from build123d import *

# Parameters (mm, degrees)
F0_W      = 127
F0_H      = 63.5
F1_DEPTH  = 177.8
F2_R      = 50.8
F3_DEPTH  = 101.6
F5_DEPTH  = 63.5
F6_R      = 19.05
F7_DEPTH  = 25.4
F9_DEPTH  = 38.1
F11_DEPTH = 38.1


with BuildPart() as f1:
    # F0 (on Front) → F1 (new body)
    with BuildSketch(Plane.XZ):
        with Locations((-4.952263087, -14.3639492443)):
            Rectangle(F0_W, F0_H)
    extrude(amount=F1_DEPTH)

    # F2 (on face) → F3 (join)
    with BuildSketch(Plane.XY.offset(17.3860507557)):
        with Locations((-4.952263087, -88.9)):
            Circle(F2_R)
    extrude(amount=F3_DEPTH)

    # F4 (on face) → F5 (cut)
    with BuildSketch(Plane.XY.offset(118.9860507557)):
        with BuildLine():
            ThreePointArc((-4.952263087, -38.1), (-30.352263087, -44.9059094878), (-48.9463535993, -63.5))
            ThreePointArc((-48.9463535993, -63.5), (-20.5993083432, -61.7985226281), (-4.952263087, -38.1))
        make_face()
        with BuildLine():
            ThreePointArc((39.0418274252, -63.5), (20.447736913, -44.9059094878), (-4.952263087, -38.1))
            ThreePointArc((-4.952263087, -38.1), (10.6947821691, -61.7985226281), (39.0418274252, -63.5))
        make_face()
        with BuildLine():
            ThreePointArc((45.847736913, -88.9), (44.1167688885, -75.7519925088), (39.0418274252, -63.5))
            ThreePointArc((39.0418274252, -63.5), (26.3418274252, -88.9), (39.0418274252, -114.3))
            ThreePointArc((39.0418274252, -114.3), (44.1167688885, -102.0480074912), (45.847736913, -88.9))
        make_face()
        with BuildLine():
            ThreePointArc((39.0418274252, -114.3), (10.6947821691, -116.0014773719), (-4.952263087, -139.7))
            ThreePointArc((-4.952263087, -139.7), (20.447736913, -132.8940905122), (39.0418274252, -114.3))
        make_face()
        with BuildLine():
            ThreePointArc((-4.952263087, -139.7), (-20.5993083432, -116.0014773719), (-48.9463535993, -114.3))
            ThreePointArc((-48.9463535993, -114.3), (-30.352263087, -132.8940905122), (-4.952263087, -139.7))
        make_face()
        with BuildLine():
            ThreePointArc((-48.9463535993, -114.3), (-36.2463535993, -88.9), (-48.9463535993, -63.5))
            ThreePointArc((-48.9463535993, -63.5), (-55.752263087, -88.9), (-48.9463535993, -114.3))
        make_face()
    extrude(amount=-F5_DEPTH, mode=Mode.SUBTRACT)

    # F6 (on face) → F7 (cut)
    with BuildSketch(Plane.XY.offset(118.9860507557)):
        with Locations((-4.952263087, -88.9)):
            Circle(F6_R)
    extrude(amount=-F7_DEPTH, mode=Mode.SUBTRACT)

    # F8 (on face) → F9 (cut)
    with BuildSketch(Plane.XY.offset(55.4860507557)):
        with BuildLine():
            ThreePointArc((-4.952263087, -139.7), (20.447736913, -132.8940905122), (39.0418274252, -114.3))
            ThreePointArc((39.0418274252, -114.3), (10.6947821691, -116.0014773719), (-4.952263087, -139.7))
        make_face()
    extrude(amount=-F9_DEPTH, mode=Mode.SUBTRACT)

    # F10 (on face) → F11 (cut)
    with BuildSketch(Plane.XY.offset(55.4860507557)):
        with BuildLine():
            Line((-4.952263087, -38.1), (39.0418274252, -63.5))
            ThreePointArc((39.0418274252, -63.5), (20.447736913, -44.9059094878), (-4.952263087, -38.1))
        make_face()
    extrude(amount=-F11_DEPTH, mode=Mode.SUBTRACT)


solid = f1.part
Could you check a few things on this model? Use its own coordinates, in mm. A direction names the side the tool comes from. Coordinates: 2 decimals unless noted, no trailing zeros. Loops run counter-clockwise (first coordinate to the right, second up) from the corner with the lowest first, then second, coordinate; pieces in that order, holes last.
1. Imagine slicing it at C-C (z = 46.5). Please give me the cut outline in (x, y), and give its area (3 significant figures).
2. For faces 5 (the face through (-20.958, -62.002, 87.681)), 6 (the face through (-36.25, -89.31, 87.68)), 7 (the face through (36, -89, 55.486)), which set-ups out of +Z, -Z, +X, -X, +Y, -Y let a thin tool reach every point of the face, with its end or its side?
3. For P1, Ø3, axis at x = -41, z = 50, coming from the -Y side; P2, Ø21.5, axis at x = -49.5, y = -92.5, coming from the +Z side; P3, Ø4, axis at x = 4, y = -88, coming from the +Z side, each with a flat end and sliding along its axis, tell me the tip position at first contact or that it passes through.
4. We'd pull the mould along X, two halves only. Please class faces 1 (the face through (16.7, -50.6, 36.7)), 2 (the face through (11.05, -115.8, 68.9)), 3 (the face through (-20.24, -116.21, 87.68)), 4 (the face through (-46, -89, 55.486)): released by +X, released by -X, zero draft, split by the parting line, or undercut.
5. I need wall thicknesses on L1, parallel to X at y = -90, z = 100.5; L2, parallel to Z at x = 33.5, y = -131; L3, parallel to Z at x = -15.5, y = -54. Which ranges of each line are inside material? Lowest first, please.
6. Imagine slicing it at D-D (x = -7.5). Please give me the cut outline in (y, z), and give its area (3 significant figures).
7. Imagine slicing it at A-A (y = -88.9). Please give me the cut outline in (x, z), and give its area (3 significant figures).
8. Imagine slicing it at B-B (x = 18). Please give me the cut outline in (y, z).
Computed values:
1. outline: (-4.95, -139.7) arc R31.75 cw to (39.04, -114.3) arc R50.8 ccw to (39.04, -63.5) - (-4.95, -38.1) arc R50.8 ccw to start
1. area: 7,190 mm2
2. face 5: +Z, +Y
2. face 6: +Z, -X
2. face 7: +Z, +X
3. P1: stops at y = -126.14
3. P2: stops at z = 55.49
3. P3: stops at z = 93.59
4. face 1: released by +X
4. face 2: undercut
4. face 3: undercut
4. face 4: zero draft
5. L1: x = -36.27 to -23.97, 14.07 to 26.36
5. L2: z = -46.11 to 17.39
5. L3: z = -46.11 to 55.49
6. outline: (-177.8, -46.11) - (0, -46.11) - (0, 17.39) - (-38.16, 17.39) - (-38.16, 55.49) - (-47.28, 55.49) - (-47.28, 118.99) - (-70.02, 118.99) - (-70.02, 93.59) - (-107.78, 93.59) - (-107.78, 118.99) - (-130.52, 118.99) - (-130.52, 55.49) - (-139.64, 55.49) - (-139.64, 17.39) - (-177.8, 17.39) - close
6. area: 19,500 mm2
7. outline: (-68.45, -46.11) - (58.55, -46.11) - (58.55, 17.39) - (45.85, 17.39) - (45.85, 55.49) - (26.34, 55.49) - (26.34, 118.99) - (14.1, 118.99) - (14.1, 93.59) - (-24, 93.59) - (-24, 118.99) - (-36.25, 118.99) - (-36.25, 55.49) - (-55.75, 55.49) - (-55.75, 17.39) - (-68.45, 17.39) - close
7. area: 14,900 mm2
8. outline: (-177.8, -46.11) - (0, -46.11) - (0, 17.39) - (-51.35, 17.39) - (-51.35, 55.49) - (-64.87, 55.49) - (-64.87, 118.99) - (-112.93, 118.99) - (-112.93, 17.39) - (-177.8, 17.39) - close
